CAD build for the part. Positions are in the model's coordinates, mm. Face numbers are marked on the shaded views. A direction names the side the tool comes from. Coordinates: 2 decimals unless noted, no trailing zeros. Loops run counter-clockwise (first coordinate to the right, second up) from the corner with the lowest first, then second, coordinate; pieces in that order, holes last. Notation, with made-up numbers: (47.25, -4) -> (94.25, -4) arc R23 ccw to (94.25, 31) -> close; hole circle Ø2 at (13, -15). An arc over 180 degrees is marked (long way). Write each question's results on one line, items separated by ' | '.
```python
from build123d import *

# Parameters (mm, degrees)
SALIENTE_EXTRUIR1_DEPTH = 200


with BuildPart() as part:
    # Croquis1 → Saliente-Extruir1 (new body)
    with BuildSketch(Plane.XY):
        Polygon((0, 0), (-59.877040429, 0), (-59.877040429, -60), (-54.877040429, -60), (-54.877040429, -10), (54.877040429, -10), (54.877040429, -60), (59.877040429, -60), (59.877040429, 0), align=None)
    extrude(amount=-SALIENTE_EXTRUIR1_DEPTH)


solid = part.part
```
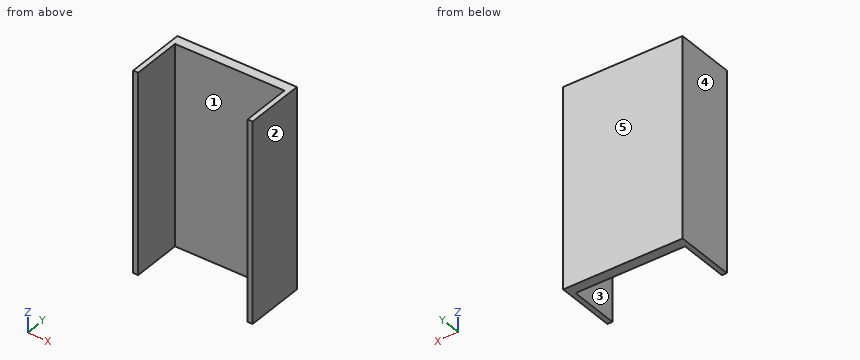
Q1. Cut at A-A on y = -31. Write the cut outline in (x, z), and give its area (3 significant figures).
Results are:
outline: (-59.88, -200) -> (-54.88, -200) -> (-54.88, 0) -> (-59.88, 0) -> close; (54.88, -200) -> (59.88, -200) -> (59.88, 0) -> (54.88, 0) -> close | area: 2,000 mm^2
Q2. Cut at C-C on x = -36. Write the cut outline in (y, z), and give its area (3 significant figures).
Results are:
outline: (-10, -200) -> (0, -200) -> (0, 0) -> (-10, 0) -> close | area: 2,000 mm^2
Q3. Pull direction X, two halves, no side cores. Call the marked faces 3, 4 and 5: +X half, -X half, draft (parallel to the pull), parting line (faces both ways), or undercut.
Results are:
face 3: undercut | face 4: -X half | face 5: draft
Q4. Which spindle directions (+Z, -Z, +X, -X, +Y, -Y) get a long thin tool onto all of the face, cutting with end or side? Do the marked faces 1 and 2. Say none if no direction does.
Results are:
face 1: +Z, -Z, -Y | face 2: +Z, -Z, +X, +Y, -Y
Q5. Drop flat-ended pins along their axis: pin 1 (2 mm diameter, centred on x = 4, z = -44.5, fed in from +Y); pin 2 (5 mm diameter, centred on x = -10, z = -72, fed in from -Y). Give the stop position or say it passes through.
Results are:
pin 1: y = 0 | pin 2: y = -10
Q6. Cut at B-B on z = -173. Write the cut outline in (x, y), and give its area (3 significant figures).
Results are:
outline: (-59.88, -60) -> (-54.88, -60) -> (-54.88, -10) -> (54.88, -10) -> (54.88, -60) -> (59.88, -60) -> (59.88, 0) -> (-59.88, 0) -> close | area: 1,700 mm^2
Q7. Wall check: L1, parallel to X at y = -27.5, z = -77; L2, parallel to Y at x = -45, z = -23. Give the ranges that are in metal, low to high. Write a range as from..to.
Results are:
L1: -59.88..-54.88, 54.88..59.88 | L2: -10..0
